```python
from build123d import *

# Parameters (mm, degrees)
F0_R     = 1.5
F0_W     = 54.5
F0_H     = 15
F1_DEPTH = 2
F2_R     = 5


with BuildPart() as f1:
    # F0 (on Top) → F1 (new body)
    with BuildSketch(Plane.XY):
        Polygon((27.25, -7.5), (33, -7.5), (33, 7.5), (-33, 7.5), (-33, -7.5), (-27.25, -7.5), align=None)
        with Locations((-30, -3.5)):
            Circle(F0_R, mode=Mode.SUBTRACT)
        with Locations((30, -3.5)):
            Circle(F0_R, mode=Mode.SUBTRACT)
        with Locations((0, -15)):
            Rectangle(F0_W, F0_H)
        with Locations((-24.25, -13.5)):
            Circle(F0_R, mode=Mode.SUBTRACT)
        with Locations((24.25, -13.5)):
            Circle(F0_R, mode=Mode.SUBTRACT)
    extrude(amount=F1_DEPTH)

    # F2
    f2_edges = [f1.edges().sort_by_distance(p)[0] for p in [
        (-33, 7.5, 1),
        (33, 7.5, 1),
        (27.25, -22.5, 1),
        (-27.25, -22.5, 1),
        (33, -7.5, 1),
        (-33, -7.5, 1),
    ]]
    fillet(f2_edges, radius=F2_R)


solid = f1.part
```
The model under review builds one solid part; all positions refer to its coordinate system, in mm. A direction names the side the tool comes from. Round coordinates to 2 decimals unless told otherwise and drop trailing zeros. Write each loop counter-clockwise with the first axis right and the second up, starting at its lowest first coordinate (ties: lowest second). Pieces come first, ordered by that corner, then holes. Notation, with made-up numbers: (30.25, -30.75) - (76.25, -30.75) arc R25 cw to (76.25, -15.75) - close; hole circle Ø2 at (33.5, 26.25). An arc over 180 degrees is marked (long way). Use one line per item in the form item = value.
Q1. Tool access review of faces 4 (the cylindrical face through (28.5, -3.43, 0.99)), 5 (the flat face through (27.25, -13, 1)), 6 (the flat face through (-27.25, -13, 1)): name each direction out of +Z, -Z, +X, -X, +Y, -Y from which nothing blocks a thin tool from reaching the whole face with its end or side.
Answer key:
face_4 = +Z, -Z
face_5 = +Z, -Z, +X, -Y
face_6 = +Z, -Z, -X, -Y
Q2. Consider section D-D (x = -24.25). State the section outline as (y, z) points, and give its area (3 significant figures).
Answer key:
outline = (-22.08, 0) - (-15, 0) - (-15, 2) - (-22.08, 2) - close; (-12, 0) - (7.5, 0) - (7.5, 2) - (-12, 2) - close
area = 53.2 mm2
Q3. Consider section C-C (x = 30). State the section outline as (y, z) points, and give its area (3 significant figures).
Answer key:
outline = (-7.08, 0) - (-5, 0) - (-5, 2) - (-7.08, 2) - close; (-2, 0) - (7.08, 0) - (7.08, 2) - (-2, 2) - close
area = 22.3 mm2
Q4. Draft analysis for pull direction X (two halves, no side actions). For faces 1 (the cylindrical face through (-31.57, -6, 1.01)), 2 (the cylindrical face through (-31.5, -3.43, 0.99)), 3 (the cylindrical face through (25.82, -21, 1.01)), state which applies: +X half, -X half, draft (parallel to the pull), parting line (faces both ways), or undercut.
Answer key:
face_1 = -X half
face_2 = undercut
face_3 = +X half
Q5. For line 1 (X direction, y = -10, z = 1.55); line 2 (X direction, y = -4, z = 1.3); line 3 (Y direction, x = 23.5, z = 0.55), list the stretches that pass through material, from the lowest coordinate up. Write a range as [from, to].
Answer key:
line_1 = [-27.25, 27.25]
line_2 = [-32.77, -31.41], [-28.59, 28.59], [31.41, 32.77]
line_3 = [-22.34, -14.8], [-12.2, 7.5]
Q6. Consider section B-B (z = 0.5). State the section outline as (x, y) points.
Answer key:
outline = (-33, -2.5) arc R5 ccw to (-28, -7.5) - (-27.25, -7.5) - (-27.25, -17.5) arc R5 ccw to (-22.25, -22.5) - (22.25, -22.5) arc R5 ccw to (27.25, -17.5) - (27.25, -7.5) - (28, -7.5) arc R5 ccw to (33, -2.5) - (33, 2.5) arc R5 ccw to (28, 7.5) - (-28, 7.5) arc R5 ccw to (-33, 2.5) - close; hole circle Ø3 at (-30, -3.5); hole circle Ø3 at (-24.25, -13.5); hole circle Ø3 at (24.25, -13.5); hole circle Ø3 at (30, -3.5)
Q7. Consider section A-A (y = -13.5). State the section outline as (x, z) points.
Answer key:
outline = (-27.25, 0) - (-25.75, 0) - (-25.75, 2) - (-27.25, 2) - close; (-22.75, 0) - (22.75, 0) - (22.75, 2) - (-22.75, 2) - close; (25.75, 0) - (27.25, 0) - (27.25, 2) - (25.75, 2) - close
